Build history of the part. All positions in model axes, mm. A direction names the side the tool comes from. Coordinates: 2 decimals unless noted, no trailing zeros. Order: outer loops, then holes, each group sorted by start corner. A loop starts at its lowest first (then second) coordinate and runs counter-clockwise, first axis right, second up. Notation, with made-up numbers: (14, -18) - (60, -18) arc R22 cw to (60, 17) - close; hole circle Ø2 at (21, 60). An arc over 180 degrees is marked (long way). Return JSON: item names as keys, results as strings.
from build123d import *

# Parameters (mm, degrees)
BOSS_EXTRUDE1_DEPTH = 50.8
SKETCH2_R           = 1.905
CUT_EXTRUDE1_DEPTH  = 101.6
CUT_EXTRUDE2_START  = -12.7
SKETCH3_R           = 5.08
CUT_EXTRUDE2_DEPTH  = 101.6
CHAMFER1_SIZE       = 3.048


with BuildPart() as part:
    # Sketch1 → Boss-Extrude1 (new body)
    with BuildSketch(Plane(origin=(0, 0, 0), x_dir=(0, 0, -1), z_dir=(1, 0, 0))):
        with BuildLine():
            Line((-61.489643294, -124.315200567), (57.124090119, -124.315200567))
            Line((57.124090119, -124.315200567), (57.124090119, -19.966735992))
            Line((57.124090119, -19.966735992), (29.562861669, -59.328249467))
            ThreePointArc((29.562861669, -59.328249467), (2.684921835, -88.660373698), (-30.868886791, -110.036507311))
            Line((-30.868886791, -110.036507311), (-61.489643294, -124.315200567))
        make_face()
    extrude(amount=BOSS_EXTRUDE1_DEPTH)

    # Sketch2 → Cut-Extrude1 (cut)
    with BuildSketch(Plane.XZ.offset(124.315200567)):
        with Locations(Location((12.7, 19.075909881, 0), (0, 0, 270))):
            Circle(SKETCH2_R)
        with Locations(Location((38.1, 19.075909881, 0), (0, 0, 270))):
            Circle(SKETCH2_R)
    extrude(amount=-CUT_EXTRUDE1_DEPTH, mode=Mode.SUBTRACT)

    # Sketch3 → Cut-Extrude2 (cut)
    with BuildSketch(Plane.XZ.offset(124.315200567).offset(CUT_EXTRUDE2_START)):
        with Locations(Location((12.7, 19.075909881, 0), (0, 0, 270))):
            Circle(SKETCH3_R)
        with Locations(Location((38.1, 19.075909881, 0), (0, 0, 270))):
            Circle(SKETCH3_R)
    extrude(amount=-CUT_EXTRUDE2_DEPTH, mode=Mode.SUBTRACT)

    # Chamfer1
    chamfer1_edges = [part.edges().sort_by_distance(p)[0] for p in [
        (12.7, -111.615200567, 24.155909881),
        (38.1, -111.615200567, 24.155909881),
    ]]
    chamfer(chamfer1_edges, length=CHAMFER1_SIZE)


solid = part.part
1. Cut at C-C on z = -19.5. Give the cut face in (x, y).
Check values:
{"outline": "(0, -124.32) - (50.8, -124.32) - (50.8, -72.18) - (0, -72.18) - close"}
2. Cut at B-B on x = 12.7. Give the cut face in (y, z), plus the area to 3 significant figures.
Check values:
{"outline": "(-124.32, -57.12) - (-19.97, -57.12) - (-59.33, -29.56) arc R152.4 cw to (-100.83, 14) - (-108.57, 14) - (-111.62, 17.04) - (-111.62, 17.17) - (-124.32, 17.17) - close; (-124.32, 20.98) - (-111.62, 20.98) - (-111.62, 21.11) - (-108.57, 24.16) - (-106.7, 24.16) arc R152.4 cw to (-110.04, 30.87) - (-124.32, 61.49) - close", "area": "4,560 mm²"}
3. Cut at A-A on x = 25.5. Give the cut face in (y, z).
Check values:
{"outline": "(-124.32, -57.12) - (-19.97, -57.12) - (-59.33, -29.56) arc R152.4 cw to (-110.04, 30.87) - (-124.32, 61.49) - close"}
4. Mould opens along Z. For faces 3 (the cylindrical face through (14.23, -105.61, 14.23)), 4 (the flat face through (25, -73, -57.124)), 5 (the flat face through (25, -124.315, 3)) say: pulls with the +Z half, pulls with the -Z half, needs draft (parallel to the pull), parting line crosses it, or undercut.
Check values:
{"face 3": "undercut", "face 4": "pulls with the -Z half", "face 5": "needs draft"}
5. Probe L1, parallel to Z at x = 12.7, y = -105; L2, parallel to Y at x = 34, z = -39; L3, parallel to Z at x = 12, y = -114. List the from-to ranges inside material, lowest first.
Check values:
{"L1": "-57.12 to 14", "L2": "-124.32 to -45.85", "L3": "-57.12 to 17.3, 20.85 to 39.37"}
6. Cut at D-D on y = -72.5. Give the cut face in (x, z), plus the area to 3 significant figures.
Check values:
{"outline": "(0, -57.12) - (50.8, -57.12) - (50.8, -19.22) - (0, -19.22) - close", "area": "1,930 mm²"}
7. Tool access for faces 1 (the cylindrical face through (25.04, -88.3, -3.11)), 2 (the cylindrical face through (36.154, -105.613, 14.383)): list every direction of +Z, -Z, +X, -X, +Y, -Y with a clear straight run to the whole face (end or side of a thin tool).
Check values:
{"face 1": "+Z, +X, -X, +Y", "face 2": "+Y"}
8. Drop flat-ended pins along their axis: pin 1 (3.5 mm diameter, centred on x = 12.5, z = 18.5, fed in from +Y); pin 2 (2.5 mm diameter, centred on x = 38.1, z = 19.08, fed in from -Y); pin 3 (2 mm diameter, centred on x = 18.5, y = -106.5, fed in from +Z); pin 4 (1 mm diameter, centred on x = 22.5, z = 24, fed in from +Y). Give the stop position or say it passes through.
Check values:
{"pin 1": "y = -111.29", "pin 2": "through", "pin 3": "z = 25.69", "pin 4": "y = -106.35"}
